Geometry check sheet. Reference: the model listing, model coordinates, mm. Round coordinates to 2 decimals unless told otherwise and drop trailing zeros. Order: outer loops, then holes, each group sorted by start corner. A loop starts at its lowest first (then second) coordinate and runs counter-clockwise, first axis right, second up.
(1) Sectioned sample at C-C (x = 170). Record the boundary of the cut face in (y, z).
(2) Material ranges on line 1 along X through (y, z) = (254, 5); line 2 along X through (y, z) = (141, 5.5); line 3 along Y through (x, z) = (198.5, 2), recorded low to high.
(3) Sectioned sample at A-A (y = 152.4). Record the boundary of the cut face in (x, z), plus the area to 3 significant figures.
(4) Sectioned sample at B-B (z = 4.75). Record the boundary of the cut face in (x, y).
(5) Go/stop test with a flat-tipped pin: pin 1 (3 mm diameter, centred on y = 142, z = 3, fed in from -X). Record where the tip stops, or that it passes through.
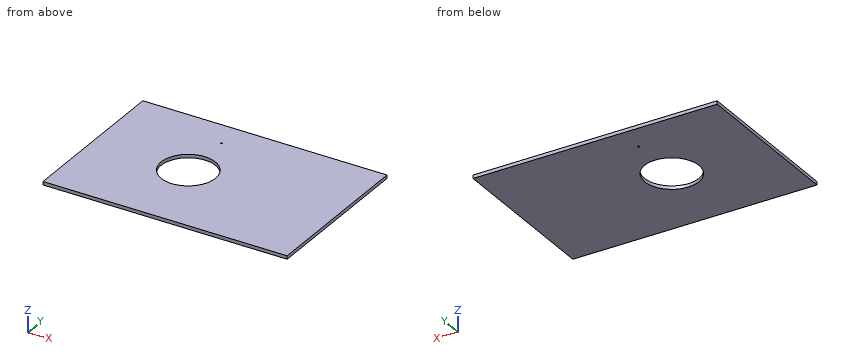
Autodesk Inventor part; units mm, degrees
ref_plane "YZ Plane" through (0, 0, 0) normal (1, 0, 0) x (0, 1, 0)
ref_plane "XZ Plane" through (0, 0, 0) normal (0, 1, 0) x (-1, 0, 0)
ref_plane "XY Plane" through (0, 0, 0) normal (0, 0, 1) x (1, 0, 0)
sketch "Sketch1" plane through (0, 0, 0) normal (0, 0, 1) x (1, 0, 0)
  line L0 (0, 0) -> (457.2, 0)
  line L1 (457.2, 0) -> (457.2, 304.8)
  line L2 (457.2, 304.8) -> (0, 304.8)
  line L3 (0, 304.8) -> (0, 0)
  arc A0 (0.6776, 254) -> (325.1105, 153.4434) centre (178.4776, 254) ccw
  circle A1 centre (178.4776, 152.4) radius 50.8
  line L4 (394.0694, 254) -> (325.1105, 153.4434)
  circle A2 centre (178.4776, 254) radius 1.4986
  line L5 (0, 254) -> (176.979, 254)
  line L6 (179.9762, 254) -> (457.2, 254)
  dimension "d0" = 457.2
  dimension "d1" = 304.8
  dimension "d4" = 101.6
sketch "Sketch2" plane through (0, 0, 0) normal (0, 0, 1) x (1, 0, 0)
  point P0 (0, 0)
extrude "Extrusion2" add sketch "Sketch1" along normal blind 6.35 contours L3 L5 A0 L4 L6 L1 L0 | L3 L2 L1 L6 A2 L5 | L5 A2 L6 L4 A0
sketch "Sketch3" plane through (0, 0, 6.35) normal (0, 0, 1) x (1, 0, 0)
  point P0 (0, 0)
properties part number "ShooterWall2"
Answer below:
1. outline: (0, 0) - (102.31, 0) - (102.31, 6.35) - (0, 6.35) - close; (202.49, 0) - (304.8, 0) - (304.8, 6.35) - (202.49, 6.35) - close
2. line 1: x = 0 to 176.98, 179.98 to 457.2
2. line 2: x = 0 to 128.97, 227.98 to 457.2
2. line 3: y = 0 to 105.71, 199.09 to 304.8
3. outline: (0, 0) - (127.68, 0) - (127.68, 6.35) - (0, 6.35) - close; (229.28, 0) - (457.2, 0) - (457.2, 6.35) - (229.28, 6.35) - close
3. area: 2,260 mm2
4. outline: (0, 0) - (457.2, 0) - (457.2, 304.8) - (0, 304.8) - close; hole circle Ø101.6 at (178.48, 152.4); hole circle Ø3 at (178.48, 254)
5. pin 1: stops at x = 0
